Here's the drawing with two shaded views (mm, measured from the low corner). I have some questions. A direction names the side the tool comes from. Round coordinates to 2 decimals unless told otherwise and drop trailing zeros. Order: outer loops, then holes, each group sorted by start corner. A loop starts at its lowest first (then second) coordinate and runs counter-clockwise, first axis right, second up.
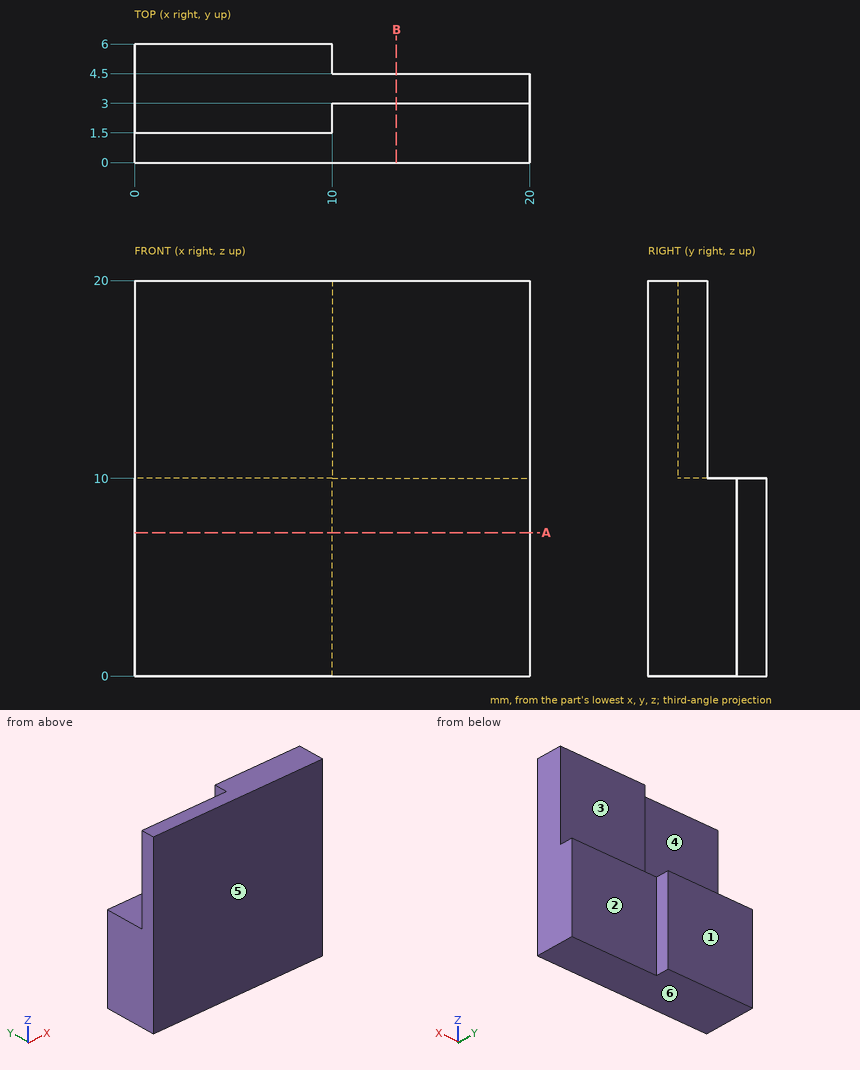
1. If we section it at A-A, the plane z = 7.25: Write out the boundary of the cut face in (x, y).
Evaluation:
outline: (0, 0) - (20, 0) - (20, 4.5) - (10, 4.5) - (10, 6) - (0, 6) - close
2. On a 3-axis mill with a long thin cutter (end or side, diameter ignored), from which of +Z, -Z, +X, -X, +Y, -Y can I reach the whole of each face in a straight line? I mean the marked faces 1, 2 and 3. Say none if no direction works.
Evaluation:
face 1: +Z, -Z, +X, -X, +Y
face 2: +Z, -Z, +X, +Y
face 3: +Z, +X, -X, +Y
3. I'm going to push flat-ended pins straight in: P1, Ø3, axis at x = 13.5, z = 15.5, coming from the +Y side; P2, Ø5, axis at x = 13, z = 5, coming from the +Y side. Where does each tip first touch, or does it pass through?
Evaluation:
P1: stops at y = 3
P2: stops at y = 4.5
4. If we section it at B-B, the plane x = 13.25: Write out the boundary of the cut face in (y, z).
Evaluation:
outline: (0, 0) - (4.5, 0) - (4.5, 10) - (3, 10) - (3, 20) - (0, 20) - close
5. If we mould it in two halves opening along Y, with no side actions, what happens to the marked faces 4, 5 and 6? For each: released by +Y, released by -Y, zero draft, split by the parting line, or undercut.
Evaluation:
face 4: released by +Y
face 5: released by -Y
face 6: zero draft
6. I need wall thicknesses on probe 1 along Z at (x, y) = (4.5, 5.35); probe 2 along Y at (x, z) = (15.75, 13.75); probe 3 along Y at (x, z) = (18.25, 4). Which ranges of each line are inside material? Lowest first, please.
Evaluation:
probe 1: z = 0 to 10
probe 2: y = 0 to 3
probe 3: y = 0 to 4.5
